The listing builds one solid part. Answer for the finished solid, in the listing's coordinates (mm). Give positions to 0.01 mm unless a question says otherwise; leave off trailing zeros. Order: outer loops, then holes, each group sorted by start corner. A loop starts at its lowest first (then second) coordinate and runs counter-clockwise, first axis right, second up. Notation, with made-up numbers: (39.25, -1) - (57.25, -1) arc R15 ccw to (57.25, 20) - close; hole circle Ø8 at (62.5, -32). An arc over 180 degrees is marked (long way). Answer in a Markdown table with one row per item.
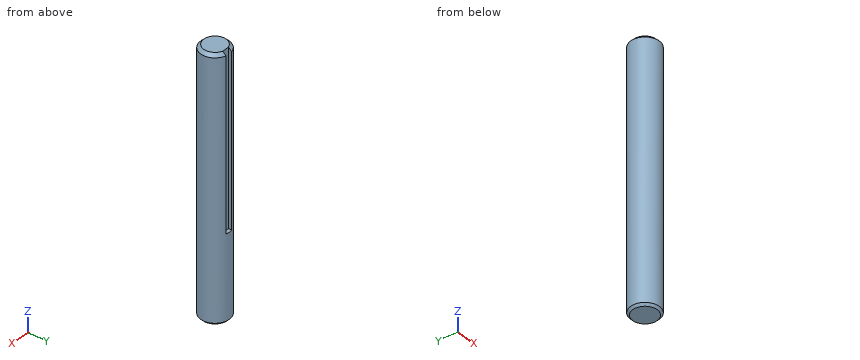
from build123d import *

# Parameters (mm, degrees)
SKETCH1_R           = 6.35
EXTRUDE1_DEPTH      = 76.2
CHAMFER1_SIZE       = 0.9525
SKETCH3_W           = 3.175
SKETCH3_H           = 1.5875
EXTRUDE2_DEPTH      = 77.727341932
EXTRUDE2_DEPTH_BACK = 38.481
CHAMFER2_SIZE       = 1.373522526


with BuildPart() as part:
    # Sketch1 → Extrude1 (new, symmetric)
    with BuildSketch(Plane.XY):
        with Locations(Location((0, 0, 0), (0, 0, 180))):
            Circle(SKETCH1_R)
    extrude(amount=EXTRUDE1_DEPTH, both=True)

    # Chamfer1
    chamfer1_edges = [part.edges().sort_by_distance(p)[0] for p in [
        (6.35, 0, -76.2),
        (6.35, 0, 76.2),
    ]]
    chamfer(chamfer1_edges, length=CHAMFER1_SIZE)

    # Sketch3 → Extrude2 (cut, two sides)
    with BuildSketch(Plane.XY) as extrude2_sk:
        with Locations((0, 5.55625)):
            Rectangle(SKETCH3_W, SKETCH3_H)
    extrude(amount=EXTRUDE2_DEPTH, mode=Mode.SUBTRACT)
    extrude(extrude2_sk.sketch, amount=-EXTRUDE2_DEPTH_BACK, mode=Mode.SUBTRACT)

    # SurfaceCut1
    split(bisect_by=Plane.XY.offset(38.1), keep=Keep.BOTTOM)

    # Chamfer2
    chamfer2_edges = [part.edges().sort_by_distance(p)[0] for p in [
        (3.888564967, -5.020115786, 38.1),
    ]]
    chamfer(chamfer2_edges, length=CHAMFER2_SIZE)


solid = part.part
Item 1: Find section C-C on z = -16. Write down the section's boundary in (x, y), then the cut area to 3 significant figures.
Answer block:
| item | result |
|---|---|
| outline | (-1.59, 4.76) - (-1.59, 6.15) arc R6.35 ccw (long way) to (1.59, 6.15) - (1.59, 4.76) - close |
| area | 122 mm² |
Item 2: Find section A-A on x = 0. Write down the section's boundary in (y, z).
Answer block:
| item | result |
|---|---|
| outline | (-6.35, -75.25) - (-5.4, -76.2) - (5.4, -76.2) - (6.35, -75.25) - (6.35, -38.48) - (4.76, -38.48) - (4.76, 38.1) - (-4.98, 38.1) - (-6.35, 36.73) - close |
Item 3: Consider line 1 (X direction, y = -0.5, z = -31); line 2 (Y direction, x = 0.25, z = -15); line 3 (Z direction, x = 5.5, y = 2.25). Determine where each line is inside the solid, lowest interval first.
Answer block:
| item | result |
|---|---|
| line 1 | -6.33 to 6.33 |
| line 2 | -6.35 to 4.76 |
| line 3 | -75.66 to 37.13 |
Item 4: Each of these flat-tipped pins is pushed along its axis until it touches: P1, Ø1, axis at x = -0.5, z = 13.5, coming from the +Y side; P2, Ø1.5, axis at y = 5.5, z = -15, coming from the -X side; P3, Ø0.8, axis at x = -0.5, y = 5.5, coming from the +Z side. Where does it stop, or does it pass through?
Answer block:
| item | result |
|---|---|
| P1 | y = 4.76 |
| P2 | x = -4.21 |
| P3 | z = -38.48 |
Item 5: Find section B-B on z = -60.5. Write down the section's boundary in (x, y), then the cut area to 3 significant figures.
Answer block:
| item | result |
|---|---|
| outline | circle Ø12.7 at (0, 0) |
| area | 127 mm² |
